from build123d import *

# Parameters (mm, degrees)
CUT_EXTRUDE1_REACH             = 18.498
SKETCH2_R                      = 3.9624
CUT_EXTRUDE1_DIRECTION_2_REACH = 18.498
F_37_0_104_DIAMETER_HOLE1_D    = 2.6416


with BuildPart() as part:
    # Sketch1 → Revolve1 (revolve)
    with BuildSketch(Plane.XY):
        with BuildLine():
            Line((-9.525, 0), (9.525, 0))
            ThreePointArc((9.525, 0), (0, 9.525), (-9.525, 0))
        make_face()
    revolve(axis=Axis((-12.682244361, 0, 0), (1, 0, 0)))

    # Sketch2 → Cut-Extrude1 (cut, up to next)
    with BuildSketch(Plane(origin=(0, 0, 0), x_dir=(0, 0, -1), z_dir=(1, 0, 0)), mode=Mode.PRIVATE) as cut_extrude1_sk1:
        with Locations(Location((0, 0, 0), (0, 0, 90))):
            Circle(SKETCH2_R)
    cut_extrude1_tool1 = extrude(cut_extrude1_sk1.sketch, amount=-CUT_EXTRUDE1_REACH, mode=Mode.PRIVATE) & part.part
    add(cut_extrude1_tool1.solids().sort_by_distance((0, 0, 0))[0], mode=Mode.SUBTRACT)

    # Sketch2 → Cut-Extrude1 direction 2 (cut, up to next)
    with BuildSketch(Plane(origin=(0, 0, 0), x_dir=(0, 0, -1), z_dir=(1, 0, 0)), mode=Mode.PRIVATE) as cut_extrude1_direction_2_sk1:
        with Locations(Location((0, 0, 0), (0, 0, 90))):
            Circle(SKETCH2_R)
    cut_extrude1_direction_2_tool1 = extrude(cut_extrude1_direction_2_sk1.sketch, amount=CUT_EXTRUDE1_DIRECTION_2_REACH, mode=Mode.PRIVATE) & part.part
    add(cut_extrude1_direction_2_tool1.solids().sort_by_distance((0, 0, 0))[0], mode=Mode.SUBTRACT)

    # #37 (0.104) Diameter Hole1 (through all)
    with Locations(Plane(origin=(0, 9.525, 0), x_dir=(1, 0, 0), z_dir=(0, 1, 0))):
        with Locations((0, 0)):
            Hole(F_37_0_104_DIAMETER_HOLE1_D / 2)


solid = part.part
Part model, mm, in its own coordinate system. Coordinates: 2 decimals unless noted, no trailing zeros. Loops run counter-clockwise (first coordinate to the right, second up) from the corner with the lowest first, then second, coordinate; pieces in that order, holes last. Notation, with made-up numbers: (1.25, 19) -> (22.25, 19) arc R19 ccw to (22.25, 41) -> close; hole circle Ø4 at (5.5, -17.5). An arc over 180 degrees is marked (long way). Use a Markdown table: item, result. Add a question column.
Item 1: Flat gauge pins, fed straight in: P1, Ø2, axis at x = 3.5, y = 5, coming from the +Z side; P2, Ø1.5, axis at x = 0, z = -2.5, coming from the -Y side; P3, Ø1.6, axis at x = 0, z = 0, coming from the +Y side (3 decimals); P4, Ø6, axis at y = 3.5, z = -6.5, coming from the -X side. Where does each tip first touch, or does it go through?
Item 2: Band-saw the part on A-A on y = 0. Write the cut outline in (x, z) (3 decimals), plus the area to 3 significant figures.
Item 3: Probe probe 1 along Z at (x, y) = (4.5, 0); probe 2 along X at (y, z) = (8, 0); probe 3 along Z at (x, y) = (0, -7). List the from-to ranges inside material, lowest first.
Item 4: Band-saw the part on D-D on y = -4.5. Write the cut outline in (x, z), plus the area to 3 significant figures.
Item 5: Band-saw the part on B-B on z = -1.75. Write the cut outline in (x, y), plus the area to 3 significant figures.
Item 6: Band-saw the part on C-C on x = -4.25. Write the cut outline in (y, z), plus the area to 3 significant figures.
Geometry says:
| question | item | result |
|---|---|---|
| 1 | P1 | z = 8.04 |
| 1 | P2 | y = -9.36 |
| 1 | P3 | through |
| 1 | P4 | x = -8.46 |
| 2 | outline | (-8.662, -3.962) arc R9.525 ccw to (8.662, -3.962) -> close; (-8.662, 3.962) -> (8.662, 3.962) arc R9.525 ccw to start |
| 2 | area | 139 mm² |
| 3 | probe 1 | -8.39 to -3.96, 3.96 to 8.39 |
| 3 | probe 2 | -5.17 to -1.32, 1.32 to 5.17 |
| 3 | probe 3 | -6.46 to -1.32, 1.32 to 6.46 |
| 4 | outline | circle Ø16.79 at (0, 0); hole circle Ø2.64 at (0, 0) |
| 4 | area | 216 mm² |
| 5 | outline | (-8.66, -3.56) arc R9.36 ccw to (8.66, -3.56) -> close; (-8.66, 3.56) -> (8.66, 3.56) arc R9.36 ccw to start |
| 5 | area | 146 mm² |
| 6 | outline | circle Ø17.05 at (0, 0); hole circle Ø7.92 at (0, 0) |
| 6 | area | 179 mm² |
